from build123d import *

# Parameters (mm, degrees)
BOSS_EXTRUDE1_DEPTH                            = 57.5
CUT_EXTRUDE1_DEPTH                             = 30
M20_TAPPED_HOLE1_D                             = 17.5
M20_TAPPED_HOLE1_DEPTH                         = 44.5
M20_TAPPED_HOLE1_TIP                           = 5.257530416491153
MIRROR2_COPY_1_DEPTH                           = 30
CUT_EXTRUDE2_DEPTH                             = 7
CUT_EXTRUDE3_DEPTH                             = 7
CBORE_START                                    = -1
CBORE_FOR_M16_HEX_SOCKET_HEAD_CAP_SC_2_R       = 8.75
CBORE_FOR_M16_HEX_SOCKET_HEAD_CAP_SCREW1_DEPTH = 34.275018433
CBORE_START_2                                  = 32
CBORE_FOR_M16_HEX_SOCKET_HEAD_CAP_SC_3_O_R     = 8.75
CBORE_FOR_M16_HEX_SOCKET_HEAD_CAP_SC_3_DEPTH   = 12.5


with BuildPart() as part:
    # Sketch1 → Boss-Extrude1 (new, symmetric)
    with BuildSketch(Plane.XY):
        Polygon((-195, 0), (195, 0), (195.00000000000003, 270), (99.9999999999997, 270.00000000000006), (2.999999999999999, 173.00000000000009), (2.999999999999999, 168.0000000000001), (-2.999999999999999, 168.0000000000001), (-2.999999999999999, 173.00000000000009), (-99.9999999999997, 270.00000000000006), (-195.00000000000003, 270), align=None)
    extrude(amount=BOSS_EXTRUDE1_DEPTH, both=True)

    # Sketch2 → Cut-Extrude1 (cut)
    with BuildSketch(Plane.XY.offset(57.5)):
        with BuildLine():
            Line((32.500000000000014, 32), (157.5, 32))
            ThreePointArc((157.5, 32), (166.33883476483186, 35.661165235168156), (170, 44.5))
            Line((170, 44.5), (170, 221.49999999999997))
            ThreePointArc((170, 221.49999999999997), (166.33883476483186, 230.3388347648318), (157.5, 234))
            Line((157.5, 234), (125.17766952966375, 233.99999999999997))
            ThreePointArc((125.17766952966375, 233.99999999999997), (120.39412662510011, 233.04849415639106), (116.3388347648319, 230.3388347648318))
            Line((116.3388347648319, 230.3388347648318), (23.661165235168177, 137.66116523516763))
            ThreePointArc((23.661165235168177, 137.66116523516763), (20.95150584360897, 133.60587337489943), (20.000000000000004, 128.82233047033586))
            Line((20.000000000000004, 128.82233047033586), (20.000000000000014, 44.5))
            ThreePointArc((20.000000000000014, 44.5), (23.66116523516817, 35.661165235168156), (32.500000000000014, 32))
        make_face()
    cut_extrude1 = extrude(amount=-CUT_EXTRUDE1_DEPTH, mode=Mode.SUBTRACT)

    # M20 Tapped Hole1
    with Locations(Plane(origin=(-1.5777e-13, 270.0000000000001, 0), x_dir=(1, 0, 0), z_dir=(0, 1, 0))):
        with Locations((-147.5, 0), (147.5, 0)):
            Hole(M20_TAPPED_HOLE1_D / 2, depth=M20_TAPPED_HOLE1_DEPTH)
            with Locations((0, 0, -(M20_TAPPED_HOLE1_DEPTH + M20_TAPPED_HOLE1_TIP / 2))):  # 118° drill point
                Cone(0, M20_TAPPED_HOLE1_D / 2, M20_TAPPED_HOLE1_TIP, mode=Mode.SUBTRACT)

    # Mirror1: Cut-Extrude1 across plane
    add(cut_extrude1.mirror(Plane(origin=(0, 0, 0), x_dir=(0, 0, 1), z_dir=(1, 0, 0))), mode=Mode.SUBTRACT)

    # Mirror2: Cut-Extrude1 across plane
    add(cut_extrude1.mirror(Plane.XY), mode=Mode.SUBTRACT)

    # Mirror2 copy 1 sketch → Mirror2 copy 1 (cut)
    with BuildSketch(Plane(origin=(0, 0, -57.5), x_dir=(-1, 0, 0), z_dir=(0, 0, -1))):
        with BuildLine():
            Line((32.500000000000014, 32), (157.5, 32))
            ThreePointArc((157.5, 32), (166.33883476483186, 35.661165235168156), (170, 44.5))
            Line((170, 44.5), (170, 221.49999999999997))
            ThreePointArc((170, 221.49999999999997), (166.33883476483186, 230.3388347648318), (157.5, 234))
            Line((157.5, 234), (125.17766952966375, 233.99999999999997))
            ThreePointArc((125.17766952966375, 233.99999999999997), (120.39412662510011, 233.04849415639106), (116.3388347648319, 230.3388347648318))
            Line((116.3388347648319, 230.3388347648318), (23.661165235168177, 137.66116523516763))
            ThreePointArc((23.661165235168177, 137.66116523516763), (20.95150584360897, 133.60587337489943), (20.000000000000004, 128.82233047033586))
            Line((20.000000000000004, 128.82233047033586), (20.000000000000014, 44.5))
            ThreePointArc((20.000000000000014, 44.5), (23.66116523516817, 35.661165235168156), (32.500000000000014, 32))
        make_face()
    extrude(amount=-MIRROR2_COPY_1_DEPTH, mode=Mode.SUBTRACT)

    # Sketch5 → Cut-Extrude2 (cut)
    with BuildSketch(Plane.XZ):
        Polygon((-11.00000000000001, -57.5), (11.00000000000001, -57.5), (11, 57.5), (-11, 57.5), align=None)
    extrude(amount=-CUT_EXTRUDE2_DEPTH, mode=Mode.SUBTRACT)

    # Sketch6 → Cut-Extrude3 (cut)
    with BuildSketch(Plane.XZ):
        Polygon((-195, -11.000000000000004), (195, -11), (195, 11), (-195, 11.000000000000004), align=None)
    extrude(amount=-CUT_EXTRUDE3_DEPTH, mode=Mode.SUBTRACT)

    # CBORE for M16 Hex Socket Head Cap Screw1: read off the stored shape, not the designer's step
    # CBORE for M16 Hex Socket Head Cap Sc 2 → CBORE for M16 Hex Socket Head Cap Screw1 (cut)
    with BuildSketch(Plane(origin=(0, 0, 0), x_dir=(1, 0, 0), z_dir=(0, 1, 0)).offset(CBORE_START)):
        with Locations((-150, -43)):
            Circle(CBORE_FOR_M16_HEX_SOCKET_HEAD_CAP_SC_2_R)
    extrude(amount=CBORE_FOR_M16_HEX_SOCKET_HEAD_CAP_SCREW1_DEPTH, mode=Mode.SUBTRACT)

    # CBORE for M16 Hex Socket Head Cap Sc 3 o → CBORE for M16 Hex Socket Head Cap Sc 3 (cut)
    with BuildSketch(Plane(origin=(0, 0, 0), x_dir=(1, 0, 0), z_dir=(0, 1, 0)).offset(CBORE_START_2)):
        with BuildLine():
            Line((-155.543924868, -31), (-157.5, -32.381619709))
            ThreePointArc((-157.5, -32.381619709), (-163, -43), (-157.5, -53.618380291))
            Line((-157.5, -53.618380291), (-155.543924868, -55))
            Line((-155.543924868, -55), (-140, -55))
            Line((-140, -55), (-140, -31))
            Line((-140, -31), (-155.543924868, -31))
        make_face()
        with Locations((-150, -43)):
            Circle(CBORE_FOR_M16_HEX_SOCKET_HEAD_CAP_SC_3_O_R, mode=Mode.SUBTRACT)
    extrude(amount=CBORE_FOR_M16_HEX_SOCKET_HEAD_CAP_SC_3_DEPTH, mode=Mode.SUBTRACT)

    # LPattern1: read off the stored shape, not the designer's step
    # LPattern1: loft between two sections, ruled curve by curve
    lpattern1_from = [
        Edge.make_three_point_arc((-157.5, 31.999999688, -53.618380291), (-163, 31.999999688, -43), (-157.5, 31.999999688, -32.381619709)),
        Edge.make_line((-157.5, 31.999999688, -32.381619709), (-157.5, 31.999999688, -53.618380291)),
    ]
    lpattern1_to = [
        Edge.make_three_point_arc((-157.5, 33.2753422, -53.618380291), (-163, 33.2753422, -43), (-157.5, 33.2753422, -32.381619709)),
        Edge.make_line((-157.5, 33.2753422, -32.381619709), (-157.5, 33.2753422, -53.618380291)),
    ]
    lpattern1 = Solid(Shell([*[Face.make_surface_from_curves(lpattern1_from[k], lpattern1_to[k]) for k in range(2)], Face(Wire(lpattern1_from)), Face(Wire(lpattern1_to))]))
    add(lpattern1, mode=Mode.SUBTRACT)

    # LPattern1 2: loft between two sections, ruled curve by curve
    lpattern1_2_from = [
        Edge.make_three_point_arc((-150, 0, -34.25), (-141.25, 0, -43), (-150, 0, -51.75)),
        Edge.make_three_point_arc((-150, 0, -51.75), (-158.75, 0, -43), (-150, 0, -34.25)),
    ]
    lpattern1_2_to = [
        Edge.make_three_point_arc((-150, 32, -34.25), (-141.25, 32, -43), (-150, 32, -51.75)),
        Edge.make_three_point_arc((-150, 32, -51.75), (-158.75, 32, -43), (-150, 32, -34.25)),
    ]
    lpattern1_2 = Solid(Shell([*[Face.make_surface_from_curves(lpattern1_2_from[k], lpattern1_2_to[k]) for k in range(2)], Face(Wire(lpattern1_2_from)), Face(Wire(lpattern1_2_to))]))
    add(lpattern1_2, mode=Mode.SUBTRACT)

    # LPattern1 3: loft between two sections, ruled curve by curve
    lpattern1_3_from = [
        Edge.make_three_point_arc((157.5, 31.999999688, 53.618380291), (163, 31.999999688, 43), (157.5, 31.999999688, 32.381619709)),
        Edge.make_line((157.5, 31.999999688, 32.381619709), (157.5, 31.999999688, 53.618380291)),
    ]
    lpattern1_3_to = [
        Edge.make_three_point_arc((157.5, 33.2753422, 53.618380291), (163, 33.2753422, 43), (157.5, 33.2753422, 32.381619709)),
        Edge.make_line((157.5, 33.2753422, 32.381619709), (157.5, 33.2753422, 53.618380291)),
    ]
    lpattern1_3 = Solid(Shell([*[Face.make_surface_from_curves(lpattern1_3_from[k], lpattern1_3_to[k]) for k in range(2)], Face(Wire(lpattern1_3_from)), Face(Wire(lpattern1_3_to))]))
    add(lpattern1_3, mode=Mode.SUBTRACT)

    # LPattern1 4: loft between two sections, ruled curve by curve
    lpattern1_4_from = [
        Edge.make_three_point_arc((150, 0, 51.75), (158.75, 0, 43), (150, 0, 34.25)),
        Edge.make_three_point_arc((150, 0, 34.25), (141.25, 0, 43), (150, 0, 51.75)),
    ]
    lpattern1_4_to = [
        Edge.make_three_point_arc((150, 32, 51.75), (158.75, 32, 43), (150, 32, 34.25)),
        Edge.make_three_point_arc((150, 32, 34.25), (141.25, 32, 43), (150, 32, 51.75)),
    ]
    lpattern1_4 = Solid(Shell([*[Face.make_surface_from_curves(lpattern1_4_from[k], lpattern1_4_to[k]) for k in range(2)], Face(Wire(lpattern1_4_from)), Face(Wire(lpattern1_4_to))]))
    add(lpattern1_4, mode=Mode.SUBTRACT)

    # LPattern1 5: loft between two sections, ruled curve by curve
    lpattern1_5_from = [
        Edge.make_three_point_arc((150, 0, -34.25), (158.75, 0, -43), (150, 0, -51.75)),
        Edge.make_three_point_arc((150, 0, -51.75), (141.25, 0, -43), (150, 0, -34.25)),
    ]
    lpattern1_5_to = [
        Edge.make_three_point_arc((150, 32, -34.25), (158.75, 32, -43), (150, 32, -51.75)),
        Edge.make_three_point_arc((150, 32, -51.75), (141.25, 32, -43), (150, 32, -34.25)),
    ]
    lpattern1_5 = Solid(Shell([*[Face.make_surface_from_curves(lpattern1_5_from[k], lpattern1_5_to[k]) for k in range(2)], Face(Wire(lpattern1_5_from)), Face(Wire(lpattern1_5_to))]))
    add(lpattern1_5, mode=Mode.SUBTRACT)

    # LPattern1 6: loft between two sections, ruled curve by curve
    lpattern1_6_from = [
        Edge.make_three_point_arc((157.5, 31.999999688, -32.381619709), (163, 31.999999688, -43), (157.5, 31.999999688, -53.618380291)),
        Edge.make_line((157.5, 31.999999688, -53.618380291), (157.5, 31.999999688, -32.381619709)),
    ]
    lpattern1_6_to = [
        Edge.make_three_point_arc((157.5, 33.2753422, -32.381619709), (163, 33.2753422, -43), (157.5, 33.2753422, -53.618380291)),
        Edge.make_line((157.5, 33.2753422, -53.618380291), (157.5, 33.2753422, -32.381619709)),
    ]
    lpattern1_6 = Solid(Shell([*[Face.make_surface_from_curves(lpattern1_6_from[k], lpattern1_6_to[k]) for k in range(2)], Face(Wire(lpattern1_6_from)), Face(Wire(lpattern1_6_to))]))
    add(lpattern1_6, mode=Mode.SUBTRACT)


solid = part.part
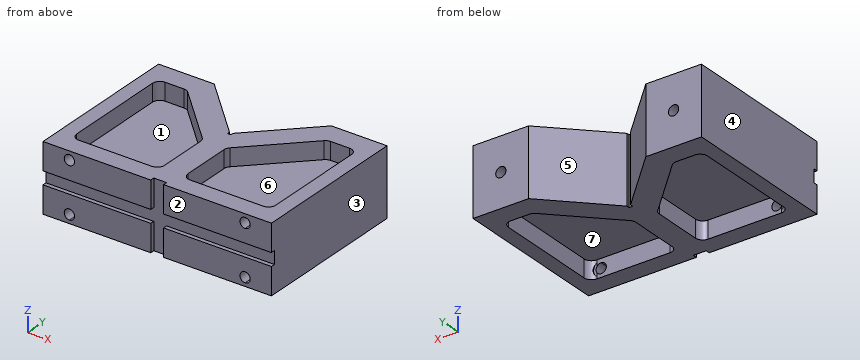
Geometry: final body of the model. Coordinates: model frame, mm. Face numbers are marked on the shaded views. A direction names the side the tool comes from. Give positions to 0.01 mm unless a question says otherwise; leave off trailing zeros. Loops run counter-clockwise (first coordinate to the right, second up) from the corner with the lowest first, then second, coordinate; pieces in that order, holes last. Notation, with made-up numbers: M 74,84 L 106,84 A19 ccw 106,118 Z; hole C 63.25,58.5 d2. An arc over 180 degrees is marked long. Put each result on its own line as item: value.
1) Cut plane C-C, the plane x = -132.5. Return the cut outline in (y, z), plus the area to 3 significant figures.
Computed values:
outline: M 0,-57.5 L 32,-57.5 L 32,-27.5 L 234,-27.5 L 234,-57.5 L 270,-57.5 L 270,57.5 L 234,57.5 L 234,27.5 L 32,27.5 L 32,57.5 L 0,57.5 L 0,11 L 7,11 L 7,-11 L 0,-11 Z
area: 18,800 mm^2
2) Cut plane D-D, the plane z = -18.5. Return the cut outline in (x, y).
Computed values:
outline: M -195,0 L -11,0 L -11,7 L 11,7 L 11,0 L 195,0 L 195,270 L 100,270 L 3,173 L 3,168 L -3,168 L -3,173 L -100,270 L -195,270 Z
3) Mould query, pull axis X, two halves, no side actions, for the marked faces 1, 2, 3 and 4. Classes: released by +X, released by -X, zero draft, split by the parting line, or undercut.
Computed values:
face 1: undercut
face 2: zero draft
face 3: released by +X
face 4: released by -X
4) Reachability of the marked faces 5, 6 and 7 from +Z, -Z, +X, -X, +Y, -Y: full face, straight path, thin tool, end or side. Return the list, or none.
Computed values:
face 5: +Z, -Z, +Y
face 6: +Z
face 7: -Z
5) Cut plane A-A, the plane y = 178.5. Return the cut outline in (x, z), plus the area to 3 significant figures.
Computed values:
outline: M -195,-57.5 L -170,-57.5 L -170,-27.5 L -64.5,-27.5 L -64.5,-57.5 L -8.5,-57.5 L -8.5,57.5 L -64.5,57.5 L -64.5,27.5 L -170,27.5 L -170,57.5 L -195,57.5 Z; M 8.5,-57.5 L 64.5,-57.5 L 64.5,-27.5 L 170,-27.5 L 170,-57.5 L 195,-57.5 L 195,57.5 L 170,57.5 L 170,27.5 L 64.5,27.5 L 64.5,57.5 L 8.5,57.5 Z
area: 30,200 mm^2
6) First-contact query: P1, Ø8, axis at x = -37.5, y = 102.5, coming from the +Z side; P2, Ø12, axis at x = -20.5, z = -38.5, coming from the +Y side; P3, Ø9, axis at x = -82.5, z = 45.5, coming from the +Y side. Flat tips, straight axial feed; report the tip coordinate or a pass-through.
Computed values:
P1: stops at z = 27.5
P2: stops at y = 196.5
P3: stops at y = 257
7) Cut plane B-B, the plane y = 248.5. Return the cut outline in (x, z).
Computed values:
outline: M -195,-57.5 L -78.5,-57.5 L -78.5,57.5 L -195,57.5 Z; M 78.5,-57.5 L 195,-57.5 L 195,57.5 L 78.5,57.5 Z; hole C -147.5,0 d17.5; hole C 147.5,0 d17.5
8) Material intervals for L1, parallel to Z at x = -150, y = 24; L2, parallel to X at y = 11.5, z = 43; L3, parallel to Z at x = -147.5, y = 253.5, sorted ascending. Write a range as from..to.
Computed values:
L1: z = -57.5..-51.75, -34.25..34.25, 51.75..57.5
L2: x = -195..-158.75, -141.25..141.25, 158.75..195
L3: z = -57.5..-8.75, 8.75..57.5
